from build123d import *

# Parameters (mm, degrees)
CROQUIS1_R              = 12.5
CROQUIS1_R_2            = 4.05
SALIENTE_EXTRUIR1_DEPTH = 20
CROQUIS2_R              = 7
CHAFL_N1_SIZE           = 6
CHAFL_N1_SIZE2          = 12
CHAFL_N2_SIZE           = 12
CHAFL_N2_SIZE2          = 6
REDONDEO1_R             = 1


with BuildPart() as part:
    # Croquis1 → Saliente-Extruir1 (new, symmetric)
    with BuildSketch(Plane.YZ):
        with Locations(Location((0, 0, 0), (0, 0, 270))):
            Circle(CROQUIS1_R)
        with Locations(Location((0, 0, 0), (0, 0, 270))):
            Circle(CROQUIS1_R_2, mode=Mode.SUBTRACT)
    extrude(amount=SALIENTE_EXTRUIR1_DEPTH, both=True)

    # Croquis2 → Cortar-Revolución1 (revolve, cut)
    with BuildSketch(Plane(origin=(0, 0, 0), x_dir=(-1, 0, 0), z_dir=(0, 1, 0)), mode=Mode.PRIVATE) as cortar_revoluci_n1_sk:
        with Locations((0, 17)):
            Circle(CROQUIS2_R)
    revolve(cortar_revoluci_n1_sk.sketch.rotate(Axis((8.275317192, 0, 0), (-1, 0, 0)), 180), axis=Axis((8.275317192, 0, 0), (-1, 0, 0)), mode=Mode.SUBTRACT)

    # Chaflán1
    chafl_n1_edges = [part.edges().sort_by_distance(p)[0] for p in [
        (-20, 0, 12.5),
    ]]
    chafl_n1_side = [part.faces().sort_by_distance(p)[0] for p in [
        (-20, 0, 12.146446609),
    ]]
    chamfer(chafl_n1_edges, length=CHAFL_N1_SIZE, length2=CHAFL_N1_SIZE2, reference=chafl_n1_side[0])

    # Chaflán2
    chafl_n2_edges = [part.edges().sort_by_distance(p)[0] for p in [
        (20, 0, 12.5),
    ]]
    chafl_n2_side = [part.faces().sort_by_distance(p)[0] for p in [
        (12.680951324, 0, 12.5),
    ]]
    chamfer(chafl_n2_edges, length=CHAFL_N2_SIZE, length2=CHAFL_N2_SIZE2, reference=chafl_n2_side[0])

    # Redondeo1
    redondeo1_edges = [part.edges().sort_by_distance(p)[0] for p in [
        (-8, 0, 12.5),
        (-20, 0, 6.5),
        (20, 0, 6.5),
        (8, 0, 12.5),
    ]]
    fillet(redondeo1_edges, radius=REDONDEO1_R)


solid = part.part
Could you check a few things on this model? Use its own coordinates, in mm. Coordinates: 2 decimals unless noted, no trailing zeros. Loops run counter-clockwise (first coordinate to the right, second up) from the corner with the lowest first, then second, coordinate; pieces in that order, holes last.
1. We'd pull the mould along Y, two halves only. Please class faces 1 (the face through (-0.28, -3.593, -1.869)), 2 (the face through (20, 4, 1.4)), 3 (the face through (-6.546, 3.755, -11.923)): released by +Y, released by -Y, zero draft, split by the parting line, or undercut.
2. Imagine slicing it at B-B (x = -3). Please give me the cut outline in (y, z).
3. For P1, Ø5, axis at x = 15, y = -3.5, coming from the +Z side; P2, Ø1, axis at x = 16, y = -3, coming from the +Z side; P3, Ø3, axis at x = -15.5, z = -4, coming from the -Y side; P4, Ø5, axis at y = 0, z = 0, coming from the -X side, each with a flat end and sliding along its axis, tell me the tip position at first contact or that it passes through.
4. I need wall thicknesses on L1, parallel to X at y = -10.25, z = -2.25; L2, parallel to X at y = 7.5, z = 7.75; L3, parallel to Y at x = -14, z = -1.5. Which ranges of each line are inside material? Lowest first, please.
5. Imagine slicing it at A-A (x = -12). Please give me the cut outline in (y, z), and give its area (3 significant figures).
Computed values:
1. face 1: undercut
1. face 2: zero draft
1. face 3: split by the parting line
2. outline: circle Ø21.35 at (0, 0); hole circle Ø8.1 at (0, 0)
3. P1: stops at z = 9.83
3. P2: stops at z = 8.27
3. P3: stops at y = -8.82
3. P4: passes through
4. L1: x = -12.01 to -2.58, 2.58 to 12.01
4. L2: x = -11.43 to -3.22, 3.22 to 11.43
4. L3: y = -9.38 to -3.76, 3.76 to 9.38
5. outline: circle Ø21 at (0, 0); hole circle Ø8.1 at (0, 0)
5. area: 295 mm2
